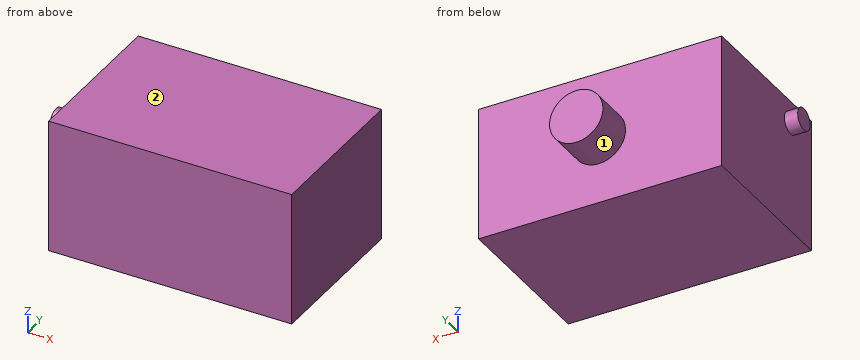
```python
from build123d import *

# Parameters (mm, degrees)
SKETCH1_W           = 91.09941719
SKETCH1_H           = 59.565003547
BOSS_EXTRUDE1_DEPTH = 50
SKETCH2_R           = 4.109340119
BOSS_EXTRUDE2_DEPTH = 5
SKETCH4_R           = 10
BOSS_EXTRUDE3_DEPTH = 15


with BuildPart() as part:
    # Sketch1 → Boss-Extrude1 (new body)
    with BuildSketch(Plane.XY):
        with Locations((-0.500546248, -0.500546249)):
            Rectangle(SKETCH1_W, SKETCH1_H)
    extrude(amount=BOSS_EXTRUDE1_DEPTH)

    # Sketch2 → Boss-Extrude2 (add)
    with BuildSketch(Plane.ZY.offset(46.050254843)):
        with Locations(Location((41.513253833, -16.406162376, 0), (0, 0, 90))):
            Circle(SKETCH2_R)
    extrude(amount=BOSS_EXTRUDE2_DEPTH)

    # Sketch4 → Boss-Extrude3 (add)
    with BuildSketch(Plane(origin=(0, 29.281955525, 0), x_dir=(1, 0, 0), z_dir=(0, 1, 0))):
        with Locations(Location((0, -25, 0), (0, 0, 270))):
            Circle(SKETCH4_R)
    extrude(amount=BOSS_EXTRUDE3_DEPTH)


solid = part.part
```
Model file for the job. Use its own axes, mm. Face numbers are marked on the shaded views. A direction names the side the tool comes from. Give positions to 0.01 mm unless a question says otherwise; leave off trailing zeros. Order: outer loops, then holes, each group sorted by start corner. A loop starts at its lowest first (then second) coordinate and runs counter-clockwise, first axis right, second up.
1) Saw through at D-D, the plane z = 11.5. Write the cut outline in (x, y), then the cut area to 3 significant figures.
2) Pin check, flat tip, straight feed: pin 1 (5 mm diameter, centred on x = -26.5, y = -11, fed in from -Z). Stop position of the tip, or through.
3) Wall check: probe 1 along X at (y, z) = (-21.5, 40.5); probe 2 along Y at (x, z) = (-14, 38); probe 3 along Z at (x, y) = (6, 31). Give the ranges that are in metal, low to high.
4) 3-axis set-ups, long thin cutter, end or side, ignore diameter. For the marked faces 1 and 2: which of +Z, -Z, +X, -X, +Y, -Y reach the whole face in a straight line?
5) Saw through at B-B, the plane z = 39. Write the cut outline in (x, y), then the cut area to 3 significant figures.
6) Saw through at C-C, the plane y = 31.5. Write the cut outline in (x, z), then the cut area to 3 significant figures.
7) Saw through at A-A, the plane x = 0. Write the cut outline in (y, z), then the cut area to 3 significant figures.
Computed:
1. outline: (-46.05, -30.28) - (45.05, -30.28) - (45.05, 29.28) - (-46.05, 29.28) - close
1. area: 5,430 mm2
2. pin 1: stops at z = 0
3. probe 1: x = -46.05 to 45.05
3. probe 2: y = -30.28 to 29.28
3. probe 3: z = 17 to 33
4. face 1: +Y
4. face 2: +Z, +X, -X, +Y, -Y
5. outline: (-51.05, -19.66) - (-46.05, -19.66) - (-46.05, -30.28) - (45.05, -30.28) - (45.05, 29.28) - (-46.05, 29.28) - (-46.05, -13.15) - (-51.05, -13.15) - close
5. area: 5,460 mm2
6. outline: circle Ø20 at (0, 25)
6. area: 314 mm2
7. outline: (-30.28, 0) - (29.28, 0) - (29.28, 15) - (44.28, 15) - (44.28, 35) - (29.28, 35) - (29.28, 50) - (-30.28, 50) - close
7. area: 3,280 mm2
